from build123d import *

# Parameters (mm, degrees)
CROQUIS1_W              = 923.8
CROQUIS1_H              = 823.8
SALIENTE_EXTRUIR1_DEPTH = 1.9
CROQUIS2_W              = 923.8
CROQUIS2_H              = 823.8
CROQUIS2_W_2            = 920
CROQUIS2_H_2            = 820
SALIENTE_EXTRUIR2_DEPTH = 25.4


with BuildPart() as part:
    # Croquis1 → Saliente-Extruir1 (new body)
    with BuildSketch(Plane(origin=(0, 0, 0), x_dir=(1, 0, 0), z_dir=(0, 1, 0))):
        Rectangle(CROQUIS1_W, CROQUIS1_H)
    extrude(amount=SALIENTE_EXTRUIR1_DEPTH)

    # Croquis2 → Saliente-Extruir2 (add)
    with BuildSketch(Plane.XZ):
        Rectangle(CROQUIS2_W, CROQUIS2_H)
        Rectangle(CROQUIS2_W_2, CROQUIS2_H_2, mode=Mode.SUBTRACT)
    extrude(amount=SALIENTE_EXTRUIR2_DEPTH)


solid = part.part
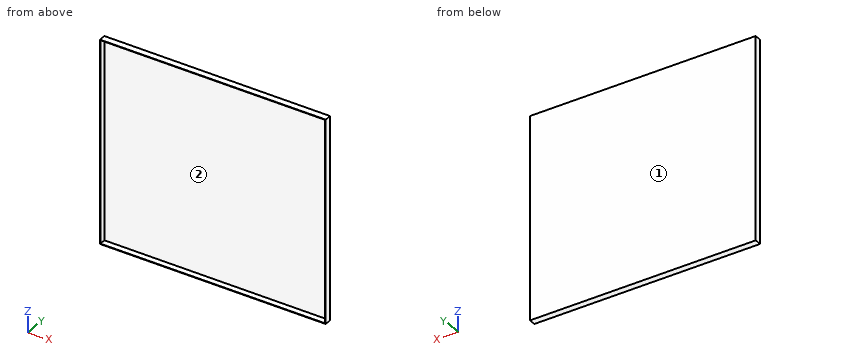
For this review, take the finished solid that the model builds, in its own axes (mm). Face numbers are marked on the shaded views. A direction names the side the tool comes from. Coordinates: 2 decimals unless noted, no trailing zeros. Write each loop counter-clockwise with the first axis right and the second up, starting at its lowest first coordinate (ties: lowest second). Pieces come first, ordered by that corner, then holes. Notation, with made-up numbers: (30.5, 68) -> (45.5, 68) arc R17 ccw to (45.5, 96) -> close; hole circle Ø8 at (4.5, 58.25). An arc over 180 degrees is marked (long way). Write each question's results on one line, items separated by ' | '. Start each with the question number.
1) For the marked faces 1 and 2, list the 3-axis set-ups (+Z, -Z, +X, -X, +Y, -Y) from which the entire face can be reached by the end or side of a thin tool; tool diameter is ignored.
2) Wall thickness on L1, parallel to Z at x = -127.5, y = -22.25; L2, parallel to X at y = -23, z = 4; L3, parallel to Y at x = -266, z = 161: over which ranges is each line inside the solid? List them lowest first. Write a range as [from, to].
3) Consider section A-A (y = -17.25). Write out the cut boundary in (x, z), plus the area to 3 significant figures.
4) Consider section C-C (x = 347). Write out the cut boundary in (y, z).
5) Consider section B-B (z = 105). Write out the cut boundary in (x, y).
Geometry says:
1) face 1: +Z, -Z, +X, -X, +Y | face 2: -Y
2) L1: [-411.9, -410], [410, 411.9] | L2: [-461.9, -460], [460, 461.9] | L3: [0, 1.9]
3) outline: (-461.9, -411.9) -> (461.9, -411.9) -> (461.9, 411.9) -> (-461.9, 411.9) -> close; hole (-460, -410) -> (460, -410) -> (460, 410) -> (-460, 410) -> close | area: 6,630 mm^2
4) outline: (-25.4, -411.9) -> (1.9, -411.9) -> (1.9, 411.9) -> (-25.4, 411.9) -> (-25.4, 410) -> (0, 410) -> (0, -410) -> (-25.4, -410) -> close
5) outline: (-461.9, -25.4) -> (-460, -25.4) -> (-460, 0) -> (460, 0) -> (460, -25.4) -> (461.9, -25.4) -> (461.9, 1.9) -> (-461.9, 1.9) -> close
